For this review, take the finished solid that the model builds, in its own axes (mm). A direction names the side the tool comes from. Give positions to 0.01 mm unless a question says otherwise; leave off trailing zeros. Order: outer loops, then holes, each group sorted by start corner. A loop starts at its lowest first (then second) coordinate and runs counter-clockwise, first axis right, second up. Notation, with made-up numbers: (83.5, -29.5) - (137.5, -29.5) arc R34 cw to (137.5, 7.5) - close; hole circle Ø7 at (-20, 68). An arc over 180 degrees is marked (long way). Use a Markdown table: item, result. Add a question column.
1) We need section A-A on y = 0. Write out the cut boundary in (x, z), then the cut area to 3 significant figures.
2) Machinability: for faces 5 (the face through (-2, 2, 262)), 6 (the face through (0, -3.9, 133)), which of the approach directions +Z, -Z, +X, -X, +Y, -Y give a long, thin tool a straight path to every point of the face, cutting with its end or side? Answer none if there is none.
3) We need section B-B on x = 0. Write out the cut boundary in (y, z).
4) Wall thickness on L1, parallel to X at y = 0, z = 208; L2, parallel to Y at x = -4.25, z = 139; L3, parallel to X at y = -5, z = 150: over which ranges is each line inside the solid? List them lowest first.
5) Clearance check with flat-ended pins moving along their axes: P1, Ø8, axis at y = 2, z = 131, coming from the -X side; P2, Ø6, axis at x = 1.5, y = 5, coming from the +Z side; P3, Ø10, axis at x = -4.5, y = 0, coming from the -Z side; P4, Ø6, axis at x = -4.5, y = 3.5, coming from the +Z side. State where each tip first meets the part, or that it passes through.
6) Mouldability with a two-part tool opening along Y and no side actions: class faces 1 (the face through (0, 3.9, 133)), 2 (the face through (-3.9, 0, 133)), 3 (the face through (-2, 2, 8)), 4 (the face through (3.9, 0, 133)) as released by +Y, released by -Y, zero draft, split by the parting line, or undercut.
```python
from build123d import *

# Parameters (mm, degrees)
SKETCH_2_R          = 2.55
EXTRUDE_1_DEPTH     = 270
CUT_EXTRUDE_1_DEPTH = 38


with BuildPart() as part:
    # 草图2 → 凸台-拉伸1 (new body)
    with BuildSketch(Plane.XY):
        with BuildLine():
            Line((-3.9, 2.839339828), (-6.560660172, 5.5))
            Line((-6.560660172, 5.5), (-8.2, 5.5))
            Line((-8.2, 5.5), (-8.2, 3.1))
            Line((-8.2, 3.1), (-9.45, 3.1))
            Line((-9.45, 3.1), (-9.45, 3.65))
            Line((-9.45, 3.65), (-10, 3.65))
            Line((-10, 3.65), (-10, 8.5))
            ThreePointArc((-10, 8.5), (-9.560660172, 9.560660172), (-8.5, 10))
            Line((-8.5, 10), (-3.65, 10))
            Line((-3.65, 10), (-3.65, 9.45))
            Line((-3.65, 9.45), (-3.1, 9.45))
            Line((-3.1, 9.45), (-3.1, 8.2))
            Line((-3.1, 8.2), (-5.5, 8.2))
            Line((-5.5, 8.2), (-5.5, 6.560660172))
            Line((-5.5, 6.560660172), (-2.839339828, 3.9))
            Line((-2.839339828, 3.9), (2.839339828, 3.9))
            Line((2.839339828, 3.9), (5.5, 6.560660172))
            Line((5.5, 6.560660172), (5.5, 8.2))
            Line((5.5, 8.2), (3.1, 8.2))
            Line((3.1, 8.2), (3.1, 9.45))
            Line((3.1, 9.45), (3.65, 9.45))
            Line((3.65, 9.45), (3.65, 10))
            Line((3.65, 10), (8.5, 10))
            ThreePointArc((8.5, 10), (9.560660172, 9.560660172), (10, 8.5))
            Line((10, 8.5), (10, 3.65))
            Line((10, 3.65), (9.45, 3.65))
            Line((9.45, 3.65), (9.45, 3.1))
            Line((9.45, 3.1), (8.2, 3.1))
            Line((8.2, 3.1), (8.2, 5.5))
            Line((8.2, 5.5), (6.560660172, 5.5))
            Line((6.560660172, 5.5), (3.9, 2.839339828))
            Line((3.9, 2.839339828), (3.9, -2.839339828))
            Line((3.9, -2.839339828), (6.560660172, -5.5))
            Line((6.560660172, -5.5), (8.2, -5.5))
            Line((8.2, -5.5), (8.2, -3.1))
            Line((8.2, -3.1), (9.45, -3.1))
            Line((9.45, -3.1), (9.45, -3.65))
            Line((9.45, -3.65), (10, -3.65))
            Line((10, -3.65), (10, -8.5))
            ThreePointArc((10, -8.5), (9.560660172, -9.560660172), (8.5, -10))
            Line((8.5, -10), (3.65, -10))
            Line((3.65, -10), (3.65, -9.45))
            Line((3.65, -9.45), (3.1, -9.45))
            Line((3.1, -9.45), (3.1, -8.2))
            Line((3.1, -8.2), (5.5, -8.2))
            Line((5.5, -8.2), (5.5, -6.560660172))
            Line((5.5, -6.560660172), (2.839339828, -3.9))
            Line((2.839339828, -3.9), (-2.839339828, -3.9))
            Line((-2.839339828, -3.9), (-5.5, -6.560660172))
            Line((-5.5, -6.560660172), (-5.5, -8.2))
            Line((-5.5, -8.2), (-3.1, -8.2))
            Line((-3.1, -8.2), (-3.1, -9.45))
            Line((-3.1, -9.45), (-3.65, -9.45))
            Line((-3.65, -9.45), (-3.65, -10))
            Line((-3.65, -10), (-8.5, -10))
            ThreePointArc((-8.5, -10), (-9.560660172, -9.560660172), (-10, -8.5))
            Line((-10, -8.5), (-10, -3.65))
            Line((-10, -3.65), (-9.45, -3.65))
            Line((-9.45, -3.65), (-9.45, -3.1))
            Line((-9.45, -3.1), (-8.2, -3.1))
            Line((-8.2, -3.1), (-8.2, -5.5))
            Line((-8.2, -5.5), (-6.560660172, -5.5))
            Line((-6.560660172, -5.5), (-3.9, -2.839339828))
            Line((-3.9, -2.839339828), (-3.9, 2.839339828))
        make_face()
        Circle(SKETCH_2_R, mode=Mode.SUBTRACT)
    extrude(amount=EXTRUDE_1_DEPTH)

    # 草图3 → 切除-拉伸1 (cut)
    with BuildSketch(Plane(origin=(0, 10, 0), x_dir=(1, 0, 0), z_dir=(0, 1, 0))):
        Polygon((-10, 0), (10, -20), (10, 0), align=None)
        Polygon((-10, -270), (10, -250), (10, -270), align=None)
    extrude(amount=-CUT_EXTRUDE_1_DEPTH, mode=Mode.SUBTRACT)


solid = part.part
```
Checked values:
| question | item | result |
|---|---|---|
| 1 | outline | (-3.9, 6.1) - (-2.55, 7.45) - (-2.55, 262.55) - (-3.9, 263.9) - close; (2.55, 12.55) - (3.9, 13.9) - (3.9, 256.1) - (2.55, 257.45) - close |
| 1 | area | 675 mm² |
| 2 | face 5 | +Z, +X, +Y, -Y |
| 2 | face 6 | +Z, -Z, -Y |
| 3 | outline | (-3.9, 10) - (-2.55, 10) - (-2.55, 260) - (-3.9, 260) - close; (2.55, 10) - (3.9, 10) - (3.9, 260) - (2.55, 260) - close |
| 4 | L1 | -3.9 to -2.55, 2.55 to 3.9 |
| 4 | L2 | -10 to -8.2, -5.31 to -3.19, 3.19 to 5.31, 8.2 to 10 |
| 4 | L3 | -10 to -8.2, -6.06 to -3.94, 3.94 to 6.06, 8.2 to 10 |
| 5 | P1 | x = -10 |
| 5 | P2 | z = 261.29 |
| 5 | P3 | z = 1.58 |
| 5 | P4 | z = 266.74 |
| 6 | face 1 | released by +Y |
| 6 | face 2 | undercut |
| 6 | face 3 | zero draft |
| 6 | face 4 | undercut |
